The model under review builds one solid part; all positions refer to its coordinate system, in mm. Face numbers are marked on the shaded views. Give positions to 0.01 mm unless a question says otherwise; leave off trailing zeros. Loops run counter-clockwise (first coordinate to the right, second up) from the corner with the lowest first, then second, coordinate; pieces in that order, holes last. Notation, with made-up numbers: M 15,-32.75 L 53,-32.75 A12 ccw 53,-13.75 Z; hole C -12.75,58.5 d1. An arc over 180 degrees is marked long. Put each result on its own line as item: value. Start each with the question number.
```python
from build123d import *

# Parameters (mm, degrees)
F0_R     = 62.5
F0_R_2   = 50
F1_DEPTH = 4
F3_DEPTH = 2


with BuildPart() as f1:
    # F0 (on Front) → F1 (new body)
    with BuildSketch(Plane.XZ):
        Circle(F0_R)
        Circle(F0_R_2, mode=Mode.SUBTRACT)
    extrude(amount=F1_DEPTH)

    # F2 (on Front) → F3 (join)
    with BuildSketch(Plane.XZ):
        Polygon((0, 0), (54.283127, 15.019991), (24.187325, 50.864834), align=None)
    extrude(amount=F3_DEPTH)


solid = f1.part
```
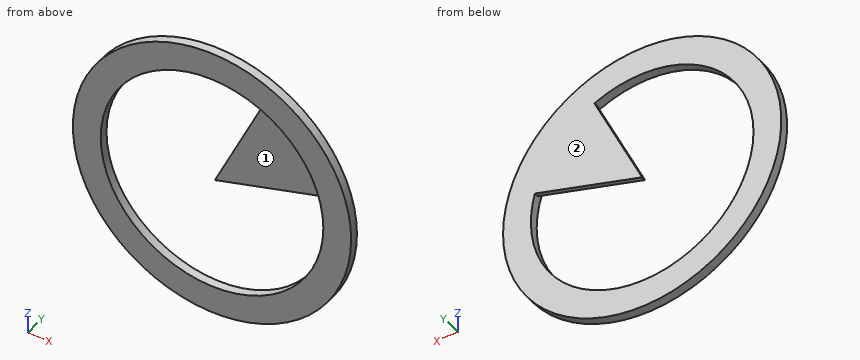
Item 1: Consider section D-D, the plane z = 36.5. Write out the cut boundary in (x, y).
Item 2: Consider section A-A, the plane x = -31. Write out the cut boundary in (y, z), plus the area to 3 significant figures.
Item 3: Consider section C-C, the plane y = -0.95. Write out the cut boundary in (x, z), plus the area to 3 significant figures.
Item 4: To check wall thickness, follow L1, parallel to Z at x = 0, y = -2.4; L2, parallel to Z at x = 3, y = -0.2; L3, parallel to Z at x = 15.5, y = -1.6. State the ranges of each line that lie inside material, in increasing order. Write a range as [from, to].
Item 5: Consider section B-B, the plane z = -48. Write out the cut boundary in (x, y).
Item 6: Draft analysis for pull direction X (two halves, no side actions). For the marked faces 1 and 2, state which applies: +X half, -X half, draft (parallel to the pull), parting line (faces both ways), or undercut.
Item 7: Clearance check with flat-ended pins moving along their axes: pin 1 Ø2 at (x, z) = (28, -43) entering from +Y; pin 2 Ø13.5 at (x, z) = (28.5, 23.5) entering from -Y; pin 3 Ø1.5 at (y, z) = (-2, 15.5) entering from +X; pin 4 Ø1.5 at (y, z) = (-1, -31.5) entering from +X. State where each tip first meets the part, or that it passes through.
Report:
1. outline: M -50.73,-4 L -34.17,-4 L -34.17,0 L -50.73,0 Z; M 17.36,-2 L 34.17,-2 L 34.17,-4 L 50.73,-4 L 50.73,0 L 17.36,0 Z
2. outline: M -4,-54.27 L 0,-54.27 L 0,-39.23 L -4,-39.23 Z; M -4,39.23 L 0,39.23 L 0,54.27 L -4,54.27 Z
2. area: 120 mm²
3. outline: C 0,0 d125; hole M 0,0 L 21.47,45.15 A50 ccw long 48.19,13.33 Z
3. area: 5,490 mm²
4. L1: [-62.5, -50], [50, 62.5]
4. L2: [-62.43, -49.91], [0.83, 6.31], [49.91, 62.43]
4. L3: [-60.55, -47.54], [4.29, 32.6], [47.54, 60.55]
5. outline: M -40.03,-4 L -14,-4 L -14,0 L -40.03,0 Z; M 14,-4 L 40.03,-4 L 40.03,0 L 14,0 Z
6. face 1: undercut
6. face 2: draft
7. pin 1: y = 0
7. pin 2: y = -2
7. pin 3: x = 60.73
7. pin 4: x = 54.41
